Drawing for the job (mm, zero at the part's lowest x, y, z). Coordinates: 2 decimals unless noted, no trailing zeros. Order: outer loops, then holes, each group sorted by start corner. A loop starts at its lowest first (then second) coordinate and runs counter-clockwise, first axis right, second up.
1) Cut at D-D (y = 16.75). List the corners of the cut face in (x, z).
2) Pin check, flat tips, straight feed: pin 1 Ø2 at (x, y) = (2.5, 3.5) entering from -Z; pin 2 Ø3 at (x, z) = (3.5, 5.5) entering from +Y. Stop position of each tip, or through.
3) Cut at A-A (x = 5). List the corners of the cut face in (y, z).
4) Mould opens along Z. For the marked faces 1, 2 and 3 say: +Z half, -Z half, draft (parallel to the pull), parting line (faces both ways), or undercut.
5) Cut at B-B (z = 8.5). List the corners of the cut face in (x, y), and give its area (3 significant figures).
6) Wall check: L1, parallel to Y at x = 3.75, z = 6; L2, parallel to X at y = 11.5, z = 6; L3, parallel to Z at x = 4.25, y = 13.5. Give the ranges that are in metal, low to high.
7) Cut at C-C (y = 6.5). List the corners of the cut face in (x, z).
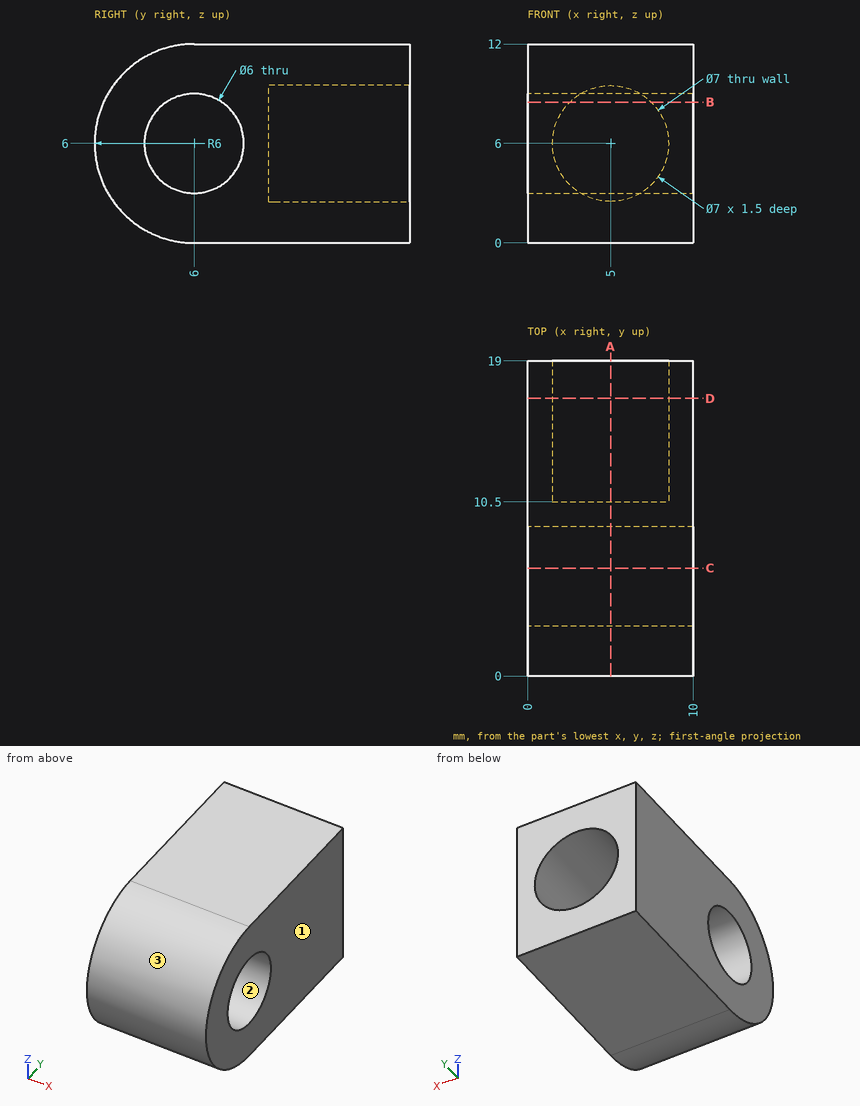
Geometry check:
1. outline: (0, 0) - (10, 0) - (10, 12) - (0, 12) - close; hole circle Ø7 at (5, 6)
2. pin 1: stops at z = 0.19
2. pin 2: stops at y = 10.5
3. outline: (6, 0) - (19, 0) - (19, 2.5) - (10.5, 2.5) - (10.5, 9.5) - (19, 9.5) - (19, 12) - (6, 12) arc R6 ccw to start; hole circle Ø6 at (6, 6)
4. face 1: draft
4. face 2: undercut
4. face 3: parting line
5. outline: (0, 0.55) - (10, 0.55) - (10, 4.34) - (0, 4.34) - close; (0, 7.66) - (10, 7.66) - (10, 19) - (7.45, 19) - (7.45, 10.5) - (2.55, 10.5) - (2.55, 19) - (0, 19) - close
5. area: 110 mm2
6. L1: y = 0 to 3, 9 to 10.5
6. L2: x = 0 to 1.5, 8.5 to 10
6. L3: z = 0 to 2.58, 9.42 to 12
7. outline: (0, 0) - (10, 0) - (10, 3.04) - (0, 3.04) - close; (0, 8.96) - (10, 8.96) - (10, 12) - (0, 12) - close
